from build123d import *

# Parameters (mm, degrees)
ESQUISSE1_W             = 13.7
ESQUISSE1_H             = 0.5
BOSS_EXTRU_1_DEPTH      = 200
ENL_V_MAT_EXTRU_1_REACH = 202.469
ESQUISSE2_R             = 1.95


with BuildPart() as part:
    # Esquisse1 → Boss.-Extru.1 (new body)
    with BuildSketch(Plane.XY):
        with Locations((6.85, 0.25)):
            Rectangle(ESQUISSE1_W, ESQUISSE1_H)
    extrude(amount=BOSS_EXTRU_1_DEPTH)

    # Esquisse2 → Enlèv. mat.-Extru.1 (cut, up to next)
    with BuildSketch(Plane(origin=(0, 0.5, 0), x_dir=(1, 0, 0), z_dir=(0, 1, 0)), mode=Mode.PRIVATE) as enl_v_mat_extru_1_sk1:
        with Locations(Location((4.5, -14.9, 0), (0, 0, 270))):
            Circle(ESQUISSE2_R)
    enl_v_mat_extru_1_tool1 = extrude(enl_v_mat_extru_1_sk1.sketch, amount=-ENL_V_MAT_EXTRU_1_REACH, mode=Mode.PRIVATE) & part.part
    # Esquisse2 → Enlèv. mat.-Extru.1 (cut, up to next)
    with BuildSketch(Plane(origin=(0, 0.5, 0), x_dir=(1, 0, 0), z_dir=(0, 1, 0)), mode=Mode.PRIVATE) as enl_v_mat_extru_1_sk2:
        with Locations(Location((4.5, -74.9, 0), (0, 0, 270))):
            Circle(ESQUISSE2_R)
    enl_v_mat_extru_1_tool2 = extrude(enl_v_mat_extru_1_sk2.sketch, amount=-ENL_V_MAT_EXTRU_1_REACH, mode=Mode.PRIVATE) & part.part
    # Esquisse2 → Enlèv. mat.-Extru.1 (cut, up to next)
    with BuildSketch(Plane(origin=(0, 0.5, 0), x_dir=(1, 0, 0), z_dir=(0, 1, 0)), mode=Mode.PRIVATE) as enl_v_mat_extru_1_sk3:
        with Locations(Location((4.5, -134.9, 0), (0, 0, 270))):
            Circle(ESQUISSE2_R)
    enl_v_mat_extru_1_tool3 = extrude(enl_v_mat_extru_1_sk3.sketch, amount=-ENL_V_MAT_EXTRU_1_REACH, mode=Mode.PRIVATE) & part.part
    # Esquisse2 → Enlèv. mat.-Extru.1 (cut, up to next)
    with BuildSketch(Plane(origin=(0, 0.5, 0), x_dir=(1, 0, 0), z_dir=(0, 1, 0)), mode=Mode.PRIVATE) as enl_v_mat_extru_1_sk4:
        with Locations(Location((4.5, -194.9, 0), (0, 0, 270))):
            Circle(ESQUISSE2_R)
    enl_v_mat_extru_1_tool4 = extrude(enl_v_mat_extru_1_sk4.sketch, amount=-ENL_V_MAT_EXTRU_1_REACH, mode=Mode.PRIVATE) & part.part
    add(enl_v_mat_extru_1_tool1.solids().sort_by_distance((4.5, 0.5, 14.9))[0], mode=Mode.SUBTRACT)
    add(enl_v_mat_extru_1_tool2.solids().sort_by_distance((4.5, 0.5, 74.9))[0], mode=Mode.SUBTRACT)
    add(enl_v_mat_extru_1_tool3.solids().sort_by_distance((4.5, 0.5, 134.9))[0], mode=Mode.SUBTRACT)
    add(enl_v_mat_extru_1_tool4.solids().sort_by_distance((4.5, 0.5, 194.9))[0], mode=Mode.SUBTRACT)


solid = part.part
CAD build for the part. Positions are in the model's coordinates, mm. Round coordinates to 2 decimals unless told otherwise and drop trailing zeros. Write each loop counter-clockwise with the first axis right and the second up, starting at its lowest first coordinate (ties: lowest second). Pieces come first, ordered by that corner, then holes. Notation, with made-up numbers: M 58.25,-34.75 L 77.25,-34.75 A23 cw 77.25,-5.75 Z; hole C -20.75,-19 d8. An arc over 180 degrees is marked long. Put each result on its own line as item: value. Start each with the question number.
1) Saw through at A-A, the plane x = 4.5. Write the cut outline in (y, z).
2) Saw through at B-B, the plane z = 14.9. Write the cut outline in (x, y), and give its area (3 significant figures).
3) Saw through at C-C, the plane y = 0.1. Write the cut outline in (x, z), and give its area (3 significant figures).
4) Drill centre lines: probe 1 along X at (y, z) = (0.2, 134.9); probe 2 along Z at (x, y) = (6, 0.2). Where is each one in solid material? Low to high. Write a range as [from, to].
5) Pull direction Z, two halves, no side cores. Call faces 1 (the flat face through (7, 0.5, 99)), 2 (the cylindrical face through (5.09, 0.25, 196.76)): pulls with the +Z half, pulls with the -Z half, needs draft (parallel to the pull), parting line crosses it, or undercut.
Resolved:
1. outline: M 0,0 L 0.5,0 L 0.5,12.95 L 0,12.95 Z; M 0,16.85 L 0.5,16.85 L 0.5,72.95 L 0,72.95 Z; M 0,76.85 L 0.5,76.85 L 0.5,132.95 L 0,132.95 Z; M 0,136.85 L 0.5,136.85 L 0.5,192.95 L 0,192.95 Z; M 0,196.85 L 0.5,196.85 L 0.5,200 L 0,200 Z
2. outline: M 0,0 L 2.55,0 L 2.55,0.5 L 0,0.5 Z; M 6.45,0 L 13.7,0 L 13.7,0.5 L 6.45,0.5 Z
2. area: 4.90 mm²
3. outline: M 0,0 L 13.7,0 L 13.7,200 L 0,200 Z; hole C 4.5,14.9 d3.9; hole C 4.5,74.9 d3.9; hole C 4.5,134.9 d3.9; hole C 4.5,194.9 d3.9
3. area: 2,690 mm²
4. probe 1: [0, 2.55], [6.45, 13.7]
4. probe 2: [0, 13.65], [16.15, 73.65], [76.15, 133.65], [136.15, 193.65], [196.15, 200]
5. face 1: needs draft
5. face 2: undercut
